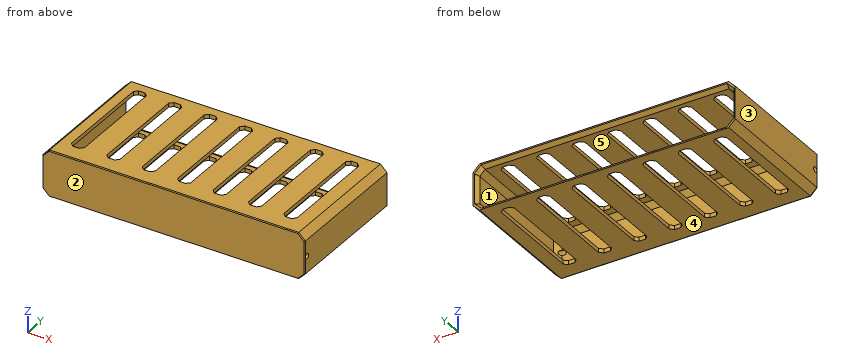
from build123d import *

# Parameters (mm, degrees)
SKETCH1_W           = 200
SKETCH1_H           = 35
SKETCH1_W_2         = 194
SKETCH1_H_2         = 29
BOSS_EXTRUDE1_DEPTH = 100
SKETCH1_3_W         = 194
SKETCH1_3_H         = 29
BOSS_EXTRUDE2_DEPTH = 3
CHAMFER1_SIZE       = 4
CHAMFER2_SIZE       = 5
CHAMFER3_SIZE       = 2
CHAMFER3_SIZE2      = 3.464101615
SKETCH2_R           = 2
CUT_EXTRUDE1_DEPTH  = 10
CHAMFER4_SIZE       = 0.5
CHAMFER4_SIZE2      = 0.866025404
CUT_EXTRUDE2_DEPTH  = 35
LPATTERN2_COUNT     = 7
LPATTERN2_PITCH     = 27


with BuildPart() as part:
    # Sketch1 → Boss-Extrude1 (new body)
    with BuildSketch(Plane(origin=(0, 0, 0), x_dir=(1, 0, 0), z_dir=(0, 1, 0))):
        Rectangle(SKETCH1_W, SKETCH1_H)
        Rectangle(SKETCH1_W_2, SKETCH1_H_2, mode=Mode.SUBTRACT)
    extrude(amount=BOSS_EXTRUDE1_DEPTH)

    # Sketch1<3> → Boss-Extrude2 (add)
    with BuildSketch(Plane(origin=(0, 0, 0), x_dir=(1, 0, 0), z_dir=(0, 1, 0))):
        Rectangle(SKETCH1_3_W, SKETCH1_3_H)
    extrude(amount=BOSS_EXTRUDE2_DEPTH)

    # Chamfer1
    chamfer1_edges = [part.edges().sort_by_distance(p)[0] for p in [
        (97, 51.5, 14.5),
        (97, 51.5, -14.5),
        (-97, 51.5, -14.5),
        (-97, 51.5, 14.5),
        (-97, 3, 0),
        (0, 3, 14.5),
        (97, 3, 0),
        (0, 3, -14.5),
    ]]
    chamfer(chamfer1_edges, length=CHAMFER1_SIZE)

    # Chamfer2
    chamfer2_edges = [part.edges().sort_by_distance(p)[0] for p in [
        (-100, 50, -17.5),
        (100, 50, -17.5),
        (100, 50, 17.5),
        (-100, 50, 17.5),
    ]]
    chamfer(chamfer2_edges, length=CHAMFER2_SIZE)

    # Chamfer3
    chamfer3_edges = [part.edges().sort_by_distance(p)[0] for p in [
        (0, 100, -14.5),
        (97, 100, 0),
        (0, 100, 14.5),
        (-97, 100, 0),
        (95, 100, -12.5),
        (95, 100, 12.5),
        (-95, 100, 12.5),
        (-95, 100, -12.5),
    ]]
    chamfer3_side = [part.faces().sort_by_distance(p)[0] for p in [
        (-97.96960595, 100, 0),
    ]]
    chamfer(chamfer3_edges, length=CHAMFER3_SIZE, length2=CHAMFER3_SIZE2, reference=chamfer3_side[0])

    # Sketch2 → Cut-Extrude1 (cut)
    with BuildSketch(Plane(origin=(100, 0, 0), x_dir=(0, 0, -1), z_dir=(1, 0, 0))):
        with Locations((0, 3)):
            Circle(SKETCH2_R)
    cut_extrude1 = extrude(amount=-CUT_EXTRUDE1_DEPTH, mode=Mode.SUBTRACT)

    # Mirror1: Cut-Extrude1 across plane
    add(cut_extrude1.mirror(Plane(origin=(0, 0, 0), x_dir=(0, 0, 1), z_dir=(1, 0, 0))), mode=Mode.SUBTRACT)

    # Chamfer4
    chamfer4_edges = [part.edges().sort_by_distance(p)[0] for p in [
        (0, 0, -17.5),
        (-100, 0, 0),
        (100, 0, 0),
        (0, 0, 17.5),
        (-97.5, 0, -15),
        (-97.5, 0, 15),
        (97.5, 0, 15),
        (97.5, 0, -15),
    ]]
    chamfer4_side = [part.faces().sort_by_distance(p)[0] for p in [
        (0, 0, 0),
    ]]
    chamfer(chamfer4_edges, length=CHAMFER4_SIZE, length2=CHAMFER4_SIZE2, reference=chamfer4_side[0])

    # Sketch3 → Cut-Extrude2 (cut)
    with BuildSketch(Plane.XY.offset(17.5)):
        Polygon((-87.421150056, 90.293329307), (-84.921150056, 92.793329307), (-79.921150056, 92.793329307), (-77.421150056, 90.293329307), (-77.421150056, 15.293329307), (-79.921150056, 12.793329307), (-84.921150056, 12.793329307), (-87.421150056, 15.293329307), align=None)
    cut_extrude2 = extrude(amount=-CUT_EXTRUDE2_DEPTH, mode=Mode.SUBTRACT)

    # LPattern2: Cut-Extrude2 ×7
    with Locations(*[(i * LPATTERN2_PITCH, 0, 0) for i in range(1, LPATTERN2_COUNT)]):
        add(cut_extrude2, mode=Mode.SUBTRACT)


solid = part.part
The listing builds one solid part. Answer for the finished solid, in the listing's coordinates (mm). Face numbers are marked on the shaded views. A direction names the side the tool comes from. Coordinates: 2 decimals unless noted, no trailing zeros. Write each loop counter-clockwise with the first axis right and the second up, starting at its lowest first coordinate (ties: lowest second). Pieces come first, ordered by that corner, then holes. Notation, with made-up numbers: (43.25, -8) - (88.25, -8) arc R26 ccw to (88.25, 15) - close; hole circle Ø5 at (-22, 8). An arc over 180 degrees is marked (long way). Answer as CSV lines item,"result".
1. Find section A-A (z = 0). Give the vertices of the cut face in (x, y).
Computed values:
outline,"(-100, 0.87) - (-99.5, 0) - (99.5, 0) - (100, 0.87) - (100, 1) - (90, 1) - (90, 3) - (-90, 3) - (-90, 1) - (-100, 1) - close; (-100, 5) - (-95, 5) - (-97, 7) - (-97, 96.54) - (-99, 100) - (-100, 100) - close; (95, 5) - (100, 5) - (100, 100) - (99, 100) - (97, 96.54) - (97, 7) - close"
2. A tool of negligible diameter and unlimited length cuts with its end or side. For the marked faces 1 and 2, from which of +Z, -Z, +X, -X, +Y, -Y can it reach the whole face along a straight path? Write none if from no direction.
Computed values:
face 1,"+Y"
face 2,"+Z, -Z, +X, -X, -Y"
3. Find section B-B (x = -18.5). Give the vertices of the cut face in (y, z), plus the area to 3 significant figures.
Computed values:
outline,"(0, -17) - (0.87, -17.5) - (100, -17.5) - (100, -16.5) - (96.54, -14.5) - (7, -14.5) - (3, -10.5) - (3, 10.5) - (7, 14.5) - (96.54, 14.5) - (100, 16.5) - (100, 17.5) - (0.87, 17.5) - (0, 17) - close"
area,"696 mm²"
4. Find section D-D (z = 8). Give the vertices of the cut face in (x, y).
Computed values:
outline,"(-100, 0.87) - (-99.5, 0) - (99.5, 0) - (100, 0.87) - (100, 100) - (99, 100) - (97, 96.54) - (97, 7) - (93, 3) - (-93, 3) - (-97, 7) - (-97, 96.54) - (-99, 100) - (-100, 100) - close"
5. Given P1, Ø0.9, axis at y = 51, z = -15.5, coming from the +X side; P2, Ø3.5, axis at x = -81.5, z = -15.5, coming from the +Y side; P3, Ø2.5, axis at y = 55, z = 15.5, coming from the -X side; P4, Ø2.5, axis at y = 57, z = 16, coming from the +X side, each flat-ended and moving along its own axis, determine where each tip first touches the part or whether it passes through.
Computed values:
P1,"stops at x = 97.45"
P2,"stops at y = 100"
P3,"stops at x = -98.25"
P4,"stops at x = 97.75"
6. Straight lines are drawn through the part: line 1 (X direction, y = 16.5, z = -4); line 2 (Z direction, x = -19.5, y = 41); line 3 (Z direction, x = 95, y = 3). For each, find the intervals that lie inside material, in ascending order. Write a range as [from, to].
Computed values:
line 1,"x = [-100, -97], [97, 100]"
line 2,"z = [-17.5, -14.5], [14.5, 17.5]"
line 3,"z = [-17.5, -2], [2, 17.5]"
7. Find section C-C (y = 56). Give the number of separate pieces and of enclosed holes in the cut face, plus the area to 3 significant figures.
Computed values:
separate pieces,"14"
enclosed holes,"0"
area,"936 mm²"
8. Determine the mould class of the marked faces 3, 4 and 5 for opening direction Z: +Z half, -Z half, draft (parallel to the pull), parting line (faces both ways), or undercut.
Computed values:
face 3,"draft"
face 4,"-Z half"
face 5,"undercut"
